from build123d import *


with BuildPart() as f1:
    # F0 (on Top) → F1 (revolve)
    with BuildSketch(Plane.XY):
        with BuildLine():
            Line((-93.137588, 47.699529), (-93.137588, 50.874529))
            Line((-93.137588, 50.874529), (-41.067588, 50.874529))
            Line((-41.067588, 50.874529), (-41.066376, 55.421129))
            Line((-41.066376, 55.421129), (-77.896376, 55.421129))
            Line((-77.896376, 55.421129), (-77.896376, 57.224529))
            Line((-77.896376, 57.224529), (-92.120376, 57.224529))
            Line((-92.120376, 57.224529), (-128.81206, 50.874529))
            ThreePointArc((-128.81206, 50.874529), (-129.540965, 50.869987), (-130.059498, 51.382282))
            Line((-130.059498, 51.382282), (-131.538478, 54.893509))
            ThreePointArc((-131.538478, 54.893509), (-135.86628, 57.135994), (-138.857588, 53.287529))
            Line((-138.857588, 53.287529), (-138.857588, 47.699529))
            Line((-138.857588, 47.699529), (-126.840025, 47.699529))
            Line((-126.840025, 47.699529), (-93.137588, 47.699529))
        make_face()
    revolve(axis=Axis((-82.501546, 44.524529, 0), (-1, 0, 0)))


solid = f1.part
Design review of the part built by this model. Coordinates are the model's own, in mm. A direction names the side the tool comes from. Coordinates: 2 decimals unless noted, no trailing zeros. Loops run counter-clockwise (first coordinate to the right, second up) from the corner with the lowest first, then second, coordinate; pieces in that order, holes last. Notation, with made-up numbers: (25, 1) -> (30, 1) arc R13 ccw to (30, 20) -> close; hole circle Ø6 at (77, 25.5). An arc over 180 degrees is marked (long way). Use a Markdown table: item, result. Add a question column.
Item 1: We need section B-B, the plane x = -94. Write out the cut boundary in (y, z) (3 decimals).
Item 2: We need section A-A, the plane z = 0. Write out the cut boundary in (x, y), and give its area (3 significant figures).
Item 3: Clearance check with flat-ended pins moving along their axes: P1, Ø6, axis at x = -95.5, y = 45.5, coming from the -Z side; P2, Ø5, axis at y = 48, z = -2.5, coming from the -X side; P3, Ø10, axis at y = 44.52, z = 0, coming from the +X side. State where each tip first meets the part, or that it passes through.
Item 4: The part is to be moulded in two halves that separate along Z. For faces 3 (the cylindrical face through (-85.108, 31.837, -0.558)), 4 (the flat face through (-77.896, 40.8, -10.4)), 5 (the flat face through (-93.138, 43, -3)), say which applies: +Z half, -Z half, draft (parallel to the pull), parting line (faces both ways), or undercut.
Item 5: Wall thickness on L1, parallel to Y at x = -82, z = 0; L2, parallel to X at y = 38.75, z = 0.5; L3, parallel to Z at x = -55.5, y = 40.5: over which ranges is each line inside the solid? List them lowest first. Write a range as from..to.
Item 6: Machinability: for faces 1 (the cylindrical face through (-60, 55, -3)), 2 (the conical face through (-130.152, 37.454, -0.311)), which of the approach directions +Z, -Z, +X, -X, +Y, -Y give a long, thin tool a straight path to every point of the face, cutting with its end or side? Answer none if there is none.
Numbers:
| question | item | result |
|---|---|---|
| 1 | outline | circle Ø24.749 at (44.525, 0); hole circle Ø6.35 at (44.525, 0) |
| 2 | outline | (-138.86, 35.76) arc R3.81 ccw to (-131.54, 34.16) -> (-130.06, 37.67) arc R0.95 cw to (-128.81, 38.17) -> (-92.12, 31.82) -> (-77.9, 31.82) -> (-77.9, 33.63) -> (-41.07, 33.63) -> (-41.07, 38.17) -> (-93.14, 38.17) -> (-93.14, 41.35) -> (-138.86, 41.35) -> close; (-138.86, 47.7) -> (-93.14, 47.7) -> (-93.14, 50.87) -> (-41.07, 50.87) -> (-41.07, 55.42) -> (-77.9, 55.42) -> (-77.9, 57.22) -> (-92.12, 57.22) -> (-128.81, 50.87) arc R0.95 cw to (-130.06, 51.38) -> (-131.54, 54.89) arc R3.81 ccw to (-138.86, 53.29) -> close |
| 2 | area | 1,130 mm^2 |
| 3 | P1 | stops at z = -12.62 |
| 3 | P2 | stops at x = -138.86 |
| 3 | P3 | stops at x = -93.14 |
| 4 | face 3 | parting line |
| 4 | face 4 | draft |
| 4 | face 5 | undercut |
| 5 | L1 | y = 31.82..38.17, 50.87..57.22 |
| 5 | L2 | x = -138.86..-93.14 |
| 5 | L3 | z = -10.13..-4.91, 4.91..10.13 |
| 6 | face 1 | +X |
| 6 | face 2 | none |
